Solid Edge part; units mm, degrees
sketch "Sketch1" plane through (0, 0, 0) normal (0, -1, 0) x (1, 0, 0)
  line L0 (9.5, 16.5) -> (9.5, -16.5)
  line L1 (13.5, -16.5) -> (9.5, -16.5)
  line L2 (13.5, -21.5) -> (13.5, -16.5)
  line L3 (22, -21.5) -> (13.5, -21.5)
  line L4 (22, -21.5) -> (22, -1.5)
  line L5 (22, -1.5) -> (38.5, -1.5)
  line L6 (38.5, -1.5) -> (38.5, 6.5)
  line L7 (38.5, 6.5) -> (15.5, 6.5)
  line L8 (15.5, 6.5) -> (15.5, 21.5)
  line L9 (15.5, 21.5) -> (13.5, 21.5)
  line L10 (13.5, 21.5) -> (13.5, 16.5)
  line L11 (13.5, 16.5) -> (9.5, 16.5)
  dimension "D1" = 38.5
  dimension "D2" = 15.5
  dimension "D3" = 13.5
  dimension "D4" = 13.5
revolve "RevolvedProtrusion1" add sketch "Sketch1" angle 360 about axis through (0, 0, 0) along (0, 0, 1)
hole "Hole1" at (0, 32.5, 6.5) direction (0, 0, -1) diameter 6.5 end up to next
pattern_circular "Pattern1" count 6 over 360 about axis through (0, 0, 6.5) along (0, 0, -1) of "Hole1"
properties part number "1976-1200-007" material "Aluminio, 7075-T6"
Source: CAD feature listing. Evaluate the final solid. Frame: model axes, mm. A direction names the side the tool comes from. Coordinates: 2 decimals unless noted, no trailing zeros. Loops run counter-clockwise (first coordinate to the right, second up) from the corner with the lowest first, then second, coordinate; pieces in that order, holes last. Notation, with made-up numbers: (28.25, -32) -> (65.25, -32) arc R6 cw to (65.25, -28) -> close; hole circle Ø9 at (-8, 29). An arc over 180 degrees is marked (long way). Answer in a Markdown table with one row per item. Add a question column.
Q1. Section D-D on x = 26.5. Return the cut outline in (y, z), and give its area (3 significant figures).
Q2. Pull-direction query (X, two-part tool) for faces 4 (the face through (-2.018, 15.368, 14.105)), 5 (the face through (-2.93, 13.18, 18.96)), 6 (the face through (17, 1, 6.5)); classes: pulls with the +X half, pulls with the -X half, needs draft (parallel to the pull), parting line crosses it, or undercut.
Q3. Section C-C on z = 15. Return the cut outline in (x, y), and give its area (3 significant figures).
Q4. Reachability of faces 1 (the face through (26.9, -19.25, 2.56)), 2 (the face through (-2.93, -13.18, -18.96)), 3 (the face through (-3.2, 9.2, 16.5)) from +Z, -Z, +X, -X, +Y, -Y: full face, straight path, thin tool, end or side. Return the list, or none.
Q5. Section A-A on x = -27. Return the cut outline in (y, z), and give its area (3 significant figures).
Q6. Section B-B on y = -32.5. Return the cut outline in (x, z), and give its area (3 significant figures).
Q7. Ray query, line 1 along Y through (x, z) = (0, 1.25); line 2 along Y through (x, z) = (0, -18.4); line 3 along X through (y, z) = (16.25, 4). Return the intervals inside material, ascending.
Q8. Contact query for flat-ended pins moving along their axis: pin 1 Ø5 at (x, z) = (20.5, -3.5) entering from -Y; pin 2 Ø4 at (x, y) = (-28.15, -16.25) entering from +Z; pin 3 Ø13.5 at (x, y) = (-2.5, 5.5) entering from +Z; pin 4 Ø8 at (x, z) = (1, 16.5) entering from -Y. Output: stop coordinate, or through.
Computed values:
| question | item | result |
|---|---|---|
| 1 | outline | (-27.93, -1.5) -> (-19.05, -1.5) -> (-19.05, 6.5) -> (-27.93, 6.5) -> close; (-13.45, -1.5) -> (13.45, -1.5) -> (13.45, 6.5) -> (-13.45, 6.5) -> close; (19.05, -1.5) -> (27.93, -1.5) -> (27.93, 6.5) -> (19.05, 6.5) -> close |
| 1 | area | 357 mm^2 |
| 2 | face 4 | parting line crosses it |
| 2 | face 5 | undercut |
| 2 | face 6 | needs draft |
| 3 | outline | circle Ø31 at (0, 0); hole circle Ø19 at (0, 0) |
| 3 | area | 471 mm^2 |
| 4 | face 1 | +Z, -Z |
| 4 | face 2 | -Z |
| 4 | face 3 | +Z |
| 5 | outline | (-27.45, -1.5) -> (-19.29, -1.5) -> (-19.29, 6.5) -> (-27.45, 6.5) -> close; (-13.21, -1.5) -> (13.21, -1.5) -> (13.21, 6.5) -> (-13.21, 6.5) -> close; (19.29, -1.5) -> (27.45, -1.5) -> (27.45, 6.5) -> (19.29, 6.5) -> close |
| 5 | area | 342 mm^2 |
| 6 | outline | (-20.64, -1.5) -> (-3.25, -1.5) -> (-3.25, 6.5) -> (-20.64, 6.5) -> close; (3.25, -1.5) -> (20.64, -1.5) -> (20.64, 6.5) -> (3.25, 6.5) -> close |
| 6 | area | 278 mm^2 |
| 7 | line 1 | y = -38.5 to -35.75, -29.25 to -9.5, 9.5 to 29.25, 35.75 to 38.5 |
| 7 | line 2 | y = -22 to -13.5, 13.5 to 22 |
| 7 | line 3 | x = -34.9 to -31.4, -24.9 to 24.9, 31.4 to 34.9 |
| 8 | pin 1 | stops at y = -33.49 |
| 8 | pin 2 | passes through |
| 8 | pin 3 | stops at z = 16.5 |
| 8 | pin 4 | stops at y = -15.5 |
